Read the model definition and answer for the solid it produces. Units are mm, in the model's axes. Face numbers are marked on the shaded views. A direction names the side the tool comes from. Give positions to 0.01 mm unless a question says otherwise; leave off trailing zeros. Loops run counter-clockwise (first coordinate to the right, second up) from the corner with the lowest first, then second, coordinate; pieces in that order, holes last.
(1) Which of the six approach directions +Z, -Z, +X, -X, +Y, -Y give full straight-line access (tool end or side, diameter ignored) to the marked faces 1, 2 and 3?
(2) Find section A-A, the plane z = 0. Write down the section's boundary in (x, y), then the cut area to 3 significant figures.
(3) Find section B-B, the plane y = -1. Write down the section's boundary in (x, z).
(4) Find section D-D, the plane x = 4. Write down the section's boundary in (y, z).
(5) Straight lines are drawn through the part: probe 1 along Z at (x, y) = (14.5, 0); probe 2 along Y at (x, z) = (16.25, -2.25); probe 3 along X at (y, z) = (0.5, -0.5). For each, find the intervals that lie inside material, in ascending order.
(6) Each of these flat-tipped pins is pushed along its axis until it touches: P1, Ø6, axis at x = 8.5, z = -4.5, coming from the +Y side; P2, Ø1, axis at x = 3.5, y = 3, coming from the +Z side; P3, Ø0.9, axis at y = -0.5, z = -0.5, coming from the +X side. Where does it stop, or does it pass through?
(7) Find section C-C, the plane x = 14.75. Write down the section's boundary in (y, z).
```python
from build123d import *

# Parameters (mm, degrees)
SKETCH_R     = 5.7
PAD_DEPTH    = 15.5
PAD001_DEPTH = 2.5
SKETCH002_R  = 1.5
POCKET_DEPTH = 5


with BuildPart() as part:
    # Sketch → Pad (new body)
    with BuildSketch(Plane.YZ):
        Circle(SKETCH_R)
    extrude(amount=PAD_DEPTH)

    # Sketch001 (on Face3 of Pad) → Pad001 (join)
    with BuildSketch(Plane.YZ.offset(15.5)):
        Polygon((0, 6), (-5.196152, 3), (-5.196152, -3), (0, -6), (5.196152, -3), (5.196152, 3), align=None)
    extrude(amount=PAD001_DEPTH)

    # Sketch002 (on Face21 of Pad001) → Pocket (cut)
    with BuildSketch(Plane.YZ.offset(18)):
        Circle(SKETCH002_R)
    extrude(amount=-POCKET_DEPTH, mode=Mode.SUBTRACT)


solid = part.part
```
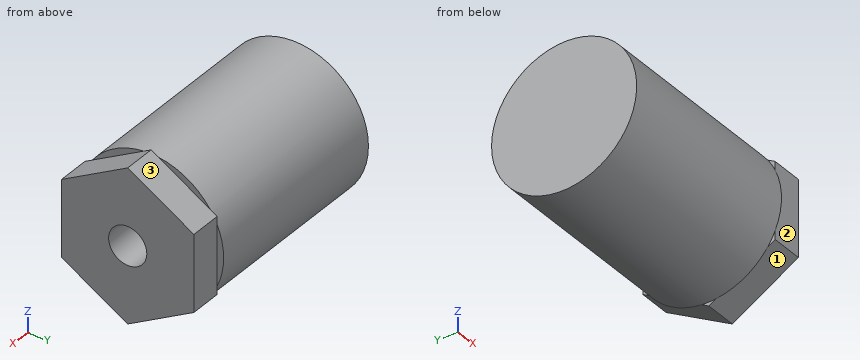
Entries:
1. face 1: -Z, +X, -Y
1. face 2: +Z, -Z, +X, -Y
1. face 3: +Z, +X, +Y
2. outline: (0, -5.7) - (15.5, -5.7) - (15.5, -5.2) - (18, -5.2) - (18, -1.5) - (13, -1.5) - (13, 1.5) - (18, 1.5) - (18, 5.2) - (15.5, 5.2) - (15.5, 5.7) - (0, 5.7) - close
2. area: 188 mm2
3. outline: (0, -5.61) - (15.5, -5.61) - (15.5, -5.42) - (18, -5.42) - (18, -1.12) - (13, -1.12) - (13, 1.12) - (18, 1.12) - (18, 5.42) - (15.5, 5.42) - (15.5, 5.61) - (0, 5.61) - close
4. outline: circle Ø11.4 at (0, 0)
5. probe 1: z = -5.7 to -1.5, 1.5 to 5.7
5. probe 2: y = -5.2 to 5.2
5. probe 3: x = 0 to 13
6. P1: stops at y = 5.5
6. P2: stops at z = 5.12
6. P3: stops at x = 13
7. outline: circle Ø11.4 at (0, 0); hole circle Ø3 at (0, 0)
